Build history of the part. All positions in model axes, mm. Face numbers are marked on the shaded views. A direction names the side the tool comes from. Round coordinates to 2 decimals unless told otherwise and drop trailing zeros. Write each loop counter-clockwise with the first axis right and the second up, starting at its lowest first coordinate (ties: lowest second). Pieces come first, ordered by that corner, then holes. Notation, with made-up numbers: (20, 12) - (25, 12) arc R7 ccw to (25, 16) - close; hole circle Ø2 at (80, 14). An arc over 180 degrees is marked (long way). Answer as a JSON object with one key per item and string values. Group by question number.
Item 1: Flat gauge pins, fed straight in: pin 1 (1 mm diameter, centred on x = -7.5, y = 5.5, fed in from +Z); pin 2 (1.5 mm diameter, centred on y = 8, z = -38.5, fed in from +X); pin 3 (2 mm diameter, centred on y = 6.5, z = 40, fed in from -X). Where does each tip first touch, or does it go through?
Item 2: Probe line 1 (Z direction, x = -33, y = 2.25); line 2 (X direction, y = 5, z = -21); line 3 (X direction, y = 5.5, z = 20). List the from-to ranges inside material, lowest first. Write a range as from..to.
Item 3: Slice it at A-A, the plane z = -28. List the corners of the cut face in (x, y) (3 decimals), then the cut area to 3 significant figures.
Item 4: Slice it at B-B, the plane x = -2. List the corners of the cut face in (y, z) (3 decimals), then the cut area to 3 significant figures.
Item 5: Which spindle directions (+Z, -Z, +X, -X, +Y, -Y) get a long thin tool onto all of the face, cutting with end or side? Do the marked faces 5, 6, 7, 8 and 9. Say none if no direction does.
Item 6: Two-plate mould, pull along Z, no slides. Class the marked faces 1, 2, 3 and 4: +Z half, -Z half, draft (parallel to the pull), parting line (faces both ways), or undercut.
Item 7: Slice it at D-D, the plane z = -4. List the corners of the cut face in (x, y) (3 decimals), then the cut area to 3 significant figures.
Item 8: Slice it at C-C, the plane y = 2. Give the number of separate pieces and of enclosed holes in the cut face, then the cut area to 3 significant figures.
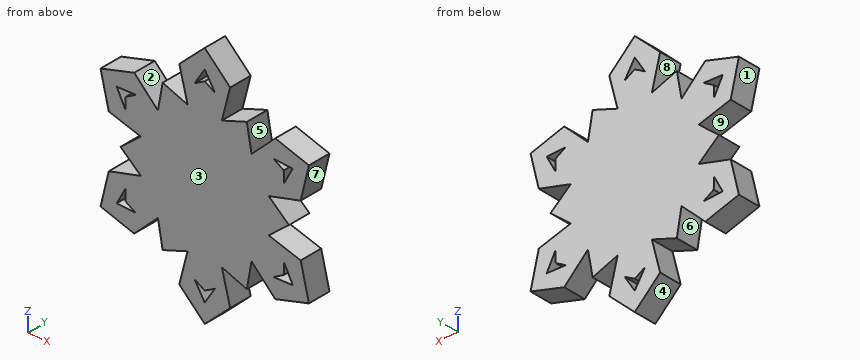
from build123d import *

# Parameters (mm, degrees)
BOSS_EXTRUDE1_DEPTH = 9.525


with BuildPart() as part:
    # Sketch1 → Boss-Extrude1 (new body)
    with BuildSketch(Plane(origin=(0, 0, 0), x_dir=(1, 0, 0), z_dir=(0, 1, 0))):
        Polygon((7.11752374, 26.562960223), (17.5, 30.310889132), (19.445436483, 19.445436483), (29.300117001, 29.120397254), (43.301270189, 25), (39.869062291, 10.81444703), (26.562960223, 7.11752374), (35, 0), (26.562960223, -7.11752374), (39.869062291, -10.81444703), (43.301270189, -25), (29.300117001, -29.120397254), (19.445436483, -19.445436483), (17.5, -30.310889132), (7.11752374, -26.562960223), (10.56894529, -39.934844284), (0, -50), (-10.56894529, -39.934844284), (-7.11752374, -26.562960223), (-17.5, -30.310889132), (-19.445436483, -19.445436483), (-29.300117001, -29.120397254), (-43.301270189, -25), (-39.869062291, -10.81444703), (-26.562960223, -7.11752374), (-35, 0), (-26.562960223, 7.11752374), (-39.869062291, 10.81444703), (-43.301270189, 25), (-29.300117001, 29.120397254), (-19.445436483, 19.445436483), (-17.5, 30.310889132), (-7.11752374, 26.562960223), (-10.56894529, 39.934844284), (0, 50), (10.56894529, 39.934844284), align=None)
        Polygon((0, 42.241346721), (4.219631638, 35.498784797), (0, 37.911261082), (-4.219631638, 35.498784797), align=None, mode=Mode.SUBTRACT)
        Polygon((28.633033619, 21.403700592), (32.832115186, 18.955630541), (32.852665257, 14.095084205), (36.58207935, 21.120673361), align=None, mode=Mode.SUBTRACT)
        Polygon((36.58207935, -21.120673361), (32.852665257, -14.095084205), (32.832115186, -18.955630541), (28.633033619, -21.403700592), align=None, mode=Mode.SUBTRACT)
        Polygon((0, -42.241346721), (4.219631638, -35.498784797), (0, -37.911261082), (-4.219631638, -35.498784797), align=None, mode=Mode.SUBTRACT)
        Polygon((-36.58207935, -21.120673361), (-28.633033619, -21.403700592), (-32.832115186, -18.955630541), (-32.852665257, -14.095084205), align=None, mode=Mode.SUBTRACT)
        Polygon((-36.58207935, 21.120673361), (-32.852665257, 14.095084205), (-32.832115186, 18.955630541), (-28.633033619, 21.403700592), align=None, mode=Mode.SUBTRACT)
    extrude(amount=BOSS_EXTRUDE1_DEPTH)


solid = part.part
Geometry says:
{
 "1": {"pin 1": "stops at z = 43.33", "pin 2": "stops at x = 10.39", "pin 3": "stops at x = -10.57"},
 "2": {"line 1": "z = -28.03..-21.25, -14.37..-8.91, -1.69..1.69, 8.91..14.37, 21.25..28.03", "line 2": "x = -42.33..-36.52, -29.33..-21.03, -19.17..19.17, 21.03..29.33, 36.52..42.33", "line 3": "x = -42.09..-35.99, -31.04..-20.01, -19.35..19.35, 20.01..31.04, 35.99..42.09"},
 "3": {"outline": "(-33.107, 0) - (-28.159, 0) - (-28.159, 9.525) - (-33.107, 9.525) - close; (-17.914, 0) - (-11.098, 0) - (-11.098, 9.525) - (-17.914, 9.525) - close; (-7.488, 0) - (7.488, 0) - (7.488, 9.525) - (-7.488, 9.525) - close; (11.098, 0) - (17.914, 0) - (17.914, 9.525) - (11.098, 9.525) - close; (28.159, 0) - (33.107, 0) - (33.107, 9.525) - (28.159, 9.525) - close", "area": "367 mm^2"},
 "4": {"outline": "(0, -48.095) - (9.525, -48.095) - (9.525, -39.046) - (0, -39.046) - close; (0, -36.768) - (9.525, -36.768) - (9.525, 36.768) - (0, 36.768) - close; (0, 39.046) - (9.525, 39.046) - (9.525, 48.095) - (0, 48.095) - close", "area": "873 mm^2"},
 "5": {"face 5": "+Z, +Y, -Y", "face 6": "-Z, +Y, -Y", "face 7": "+X, +Y, -Y", "face 8": "+Y, -Y", "face 9": "-X, +Y, -Y"},
 "6": {"face 1": "undercut", "face 2": "+Z half", "face 3": "draft", "face 4": "-Z half"},
 "7": {"outline": "(-30.258, 0) - (30.258, 0) - (30.258, 9.525) - (-30.258, 9.525) - close", "area": "576 mm^2"},
 "8": {"separate pieces": "1", "enclosed holes": "6", "area": "4,580 mm^2"}
}
